```python
from build123d import *

# Parameters (mm, degrees)
F0_W           = 8.89
F0_H           = 15.24
F1_DEPTH       = 22.86
F3_DEPTH       = 25.4
F3_DEPTH_BACK  = 25.4
F4_R           = 4.2926
F6_DEPTH       = 25.4
F6_DEPTH_BACK  = 25.4
F7_R           = 4.2924717139
F9_DEPTH       = 25.4
F9_DEPTH_BACK  = 25.4
F10_R          = 9.8901735715
F11_DEPTH      = 48.514
F12_R          = 2.8768000524
F13_DEPTH      = 25.4
F13_DEPTH_BACK = 25.4
F15_DEPTH      = 25.4
F15_DEPTH_BACK = 25.4
F16_W          = 8.89
F16_H          = 15.1638
F17_DEPTH      = 3.0734
F18_R          = 16.0782
F19_DEPTH      = 25.4
F19_DEPTH_BACK = 25.4


with BuildPart() as f1:
    # F0 (on Top) → F1 (new body)
    with BuildSketch(Plane.XY):
        Rectangle(F0_W, F0_H)
    extrude(amount=F1_DEPTH)

    # F2 (on Right) → F3 (cut, two sides)
    with BuildSketch(Plane.YZ) as f3_sk:
        Polygon((7.8410664573, 2.7272452135), (7.8410664573, 0), (12.4911786988, 0), (12.4911786988, 24.5470050722), (5.1583079621, 24.5470050722), (5.1583079621, 2.7272452135), align=None)
    extrude(amount=-F3_DEPTH, mode=Mode.SUBTRACT)
    extrude(f3_sk.sketch, amount=F3_DEPTH_BACK, mode=Mode.SUBTRACT)

    # F4
    f4_edges = [f1.edges().sort_by_distance(p)[0] for p in [
        (0, 5.158308, 22.86),
    ]]
    fillet(f4_edges, radius=F4_R)

    # F5 (on Right) → F6 (cut, two sides)
    with BuildSketch(Plane.YZ) as f6_sk:
        Polygon((-11.5864574909, 8.9812148362), (-9.2614004388, 8.9812148362), (-3.9853109047, 8.9812148362), (-3.9853109047, 24.7200578451), (-11.5864574909, 24.7200578451), align=None)
    extrude(amount=-F6_DEPTH, mode=Mode.SUBTRACT)
    extrude(f6_sk.sketch, amount=F6_DEPTH_BACK, mode=Mode.SUBTRACT)

    # F7
    f7_edges = [f1.edges().sort_by_distance(p)[0] for p in [
        (0, -3.985311, 22.86),
    ]]
    fillet(f7_edges, radius=F7_R)

    # F8 (on Right) → F9 (cut, two sides)
    with BuildSketch(Plane.YZ) as f9_sk:
        with BuildLine():
            Line((-5.4170731455, 3.8172584027), (-5.4170731455, 10.038449429))
            Line((-5.4170731455, 10.038449429), (-13.4461307898, 9.9321035668))
            Line((-13.4461307898, 9.9321035668), (-13.4461307898, 0.467386446))
            add(Edge.make_bspline(
                [(-5.4170731455, 3.8172584027), (-5.523418542, 2.6474618353), (-5.4771876546, 2.0387220808), (-7.508362437, -0.9482839925), (-11.1789391189, -0.0271654713), (-13.4461307898, 0.467386446)],
                knots=[0, 0, 0, 0, 0.2588835968, 0.5538040318, 1, 1, 1, 1], degree=3))
        make_face()
    extrude(amount=-F9_DEPTH, mode=Mode.SUBTRACT)
    extrude(f9_sk.sketch, amount=F9_DEPTH_BACK, mode=Mode.SUBTRACT)

    # F10 (on Top) → F11 (cut)
    with BuildSketch(Plane.XY):
        with Locations((0, 16.5352746844)):
            Circle(F10_R)
    extrude(amount=F11_DEPTH, mode=Mode.SUBTRACT)

    # F12 (on Front) → F13 (cut, two sides)
    with BuildSketch(Plane.XZ) as f13_sk:
        with Locations((0, 6.9304113276)):
            Circle(F12_R)
    extrude(amount=-F13_DEPTH, mode=Mode.SUBTRACT)
    extrude(f13_sk.sketch, amount=F13_DEPTH_BACK, mode=Mode.SUBTRACT)

    # F14 (on Front) → F15 (cut, two sides)
    with BuildSketch(Plane.XZ) as f15_sk:
        Polygon((-2.8829, 6.8600848975), (0, 6.8600848975), (0, 23.8157852443), (-2.8829, 24.1923942218), align=None)
        Polygon((0, 6.8600848975), (2.8829, 6.8600848975), (2.8829, 24.0822033214), (-1.0464692745, 24.0822033214), (0, 23.8157852443), align=None)
    extrude(amount=-F15_DEPTH, mode=Mode.SUBTRACT)
    extrude(f15_sk.sketch, amount=F15_DEPTH_BACK, mode=Mode.SUBTRACT)

    # F16 (on Top) → F17 (join)
    with BuildSketch(Plane.XY):
        Rectangle(F16_W, F16_H)
    extrude(amount=-F17_DEPTH)

    # F18 (on Front) → F19 (cut, two sides)
    with BuildSketch(Plane.XZ) as f19_sk:
        with Locations((0, -18.5737498105)):
            Circle(F18_R)
    extrude(amount=-F19_DEPTH, mode=Mode.SUBTRACT)
    extrude(f19_sk.sketch, amount=F19_DEPTH_BACK, mode=Mode.SUBTRACT)


solid = f1.part
```
The listing builds one solid part. Answer for the finished solid, in the listing's coordinates (mm). A direction names the side the tool comes from. Round coordinates to 2 decimals unless told otherwise and drop trailing zeros. Loops run counter-clockwise (first coordinate to the right, second up) from the corner with the lowest first, then second, coordinate; pieces in that order, holes last. Notation, with made-up numbers: (75.5, 59) - (129.5, 59) arc R24 cw to (129.5, 71) - close; hole circle Ø6 at (38, -19.5). An arc over 180 degrees is marked (long way). Return JSON: item names as keys, results as strings. Group by question number.
1. The mould has two halves that part along X. Classify faces 1 (the flat face through (-4.445, 0, 10)), 2 (the flat face through (4.445, 0, 10)), 3 (the cylindrical face through (-0.062, -0.055, 4.054)), 4 (the cylindrical face through (-3.65, -2.76, 21.57)): pulls with the +X half, pulls with the -X half, needs draft (parallel to the pull), parting line crosses it, or undercut.
2. The part is cut by section C-C on z = 10.5. Determine the outline of the cut face in (x, y) (3 decimals), then the cut area to 3 significant figures.
3. The part is cut by section A-A on z = 7.75. Determine the outline of the cut face in (x, y) (3 decimals).
4. Which of the six approach directions +Z, -Z, +X, -X, +Y, -Y give full straight-line access (tool end or side, diameter ignored) to faces 5 (the flat face through (-4, -3.985, 14)), 6 (the cylindrical face through (-0.062, 6.645, 1.345)), 7 (the cylindrical face through (-3.653, 3.867, 21.636)), 8 (the cylindrical face through (0.061, 0.106, -2.496)), 9 (the flat face through (2.883, 0, 15))?
5. Each of these flat-tipped pins is pushed along its axis until it touches: P1, Ø1.7, axis at x = -3.5, z = 14.5, coming from the -Y side; P2, Ø0.9, axis at x = 1, z = -1.5, coming from the +Y side; P3, Ø1.5, axis at x = 2, y = 0.5, coming from the -Z side. Where does it stop, or does it pass through?
6. The part is cut by section D-D on y = -0.25. Determine the outline of the cut face in (x, z) (3 decimals), then the cut area to 3 significant figures.
7. The part is cut by section B-B on y = -3.25. Determine the outline of the cut face in (x, z) (3 decimals), then the cut area to 3 significant figures.
8. Consider probe 1 along X at (y, z) = (-2.5, 10) (3 decimals); probe 2 along Y at (x, z) = (4.25, 18.5); probe 3 along Y at (x, z) = (2.75, -1.75). Determine where each line is inside the solid, lowest interval first.
Resolved:
{
 "1": {"face 1": "pulls with the -X half", "face 2": "pulls with the +X half", "face 3": "undercut", "face 4": "needs draft"},
 "2": {"outline": "(-4.445, -3.985) - (-2.883, -3.985) - (-2.883, 5.158) - (-4.445, 5.158) - close; (2.883, -3.985) - (4.445, -3.985) - (4.445, 5.158) - (2.883, 5.158) - close", "area": "28.6 mm²"},
 "3": {"outline": "(-4.445, -5.417) - (-2.883, -5.417) - (-2.883, 5.158) - (-4.445, 5.158) - close; (2.883, -5.417) - (4.445, -5.417) - (4.445, 5.158) - (2.883, 5.158) - close"},
 "4": {"face 5": "+Z, +X, -X, -Y", "face 6": "+Z, +Y", "face 7": "+Z, +X, -X, +Y", "face 8": "-Z, +Y, -Y", "face 9": "+Z, +Y, -Y"},
 "5": {"P1": "stops at y = -3.99", "P2": "stops at y = 7.58", "P3": "stops at z = -2.73"},
 "6": {"outline": "(-4.445, -3.073) - (-4.272, -3.073) arc R16.078 cw to (4.272, -3.073) - (4.445, -3.073) - (4.445, 22.824) - (2.883, 22.824) - (2.883, 6.86) - (2.876, 6.86) arc R2.877 cw to (-2.876, 6.86) - (-2.883, 6.86) - (-2.883, 22.824) - (-4.445, 22.824) - close", "area": "122 mm²"},
 "7": {"outline": "(-4.445, -3.073) - (-4.272, -3.073) arc R16.078 cw to (4.272, -3.073) - (4.445, -3.073) - (4.445, 20.97) - (2.883, 20.97) - (2.883, 6.86) - (2.876, 6.86) arc R2.877 cw to (-2.876, 6.86) - (-2.883, 6.86) - (-2.883, 20.97) - (-4.445, 20.97) - close", "area": "116 mm²"},
 "8": {"probe 1": "x = -4.445 to -2.883, 2.883 to 4.445", "probe 2": "y = -3.99 to 5.16", "probe 3": "y = -7.58 to 7.58"}
}
